For this review, take the finished solid that the model builds, in its own axes (mm). A direction names the side the tool comes from. Round coordinates to 2 decimals unless told otherwise and drop trailing zeros. Loops run counter-clockwise (first coordinate to the right, second up) from the corner with the lowest first, then second, coordinate; pieces in that order, holes last.
1) Wall thickness on L1, parallel to X at y = -1, z = -0.15; L2, parallel to X at y = -0.5, z = -0.4; L3, parallel to Z at x = 0.75, y = 0.75: over which ranges is each line inside the solid? List them lowest first.
2) Mouldability with a two-part tool opening along X and no side actions: class faces 3 (the flat face through (0, 4.674, -2)), 4 (the cylindrical face through (0.45, 0.5, 1.43)), 5 (the cylindrical face through (1.55, -3.15, -0.81)) as pulls with the +X half, pulls with the -X half, needs draft (parallel to the pull), parting line crosses it, or undercut.
3) Insertion check: pin 1 (3 mm diameter, centred on x = 0.5, y = 3.5, fed in from +Z); pin 2 (3 mm diameter, centred on x = 2, z = 2, fed in from -Y). Each pin has a flat end and moves straight along its axis. Give the tip position at first contact, or say it passes through.
4) Tool access review of faces 1 (the conical face through (1.9, 3.07, 0.42)), 2 (the flat face through (1.2, -3.8, -1.2)): name each direction out of +Z, -Z, +X, -X, +Y, -Y from which nothing blocks a thin tool from reaching the whole face with its end or side.
5) Take a section at B-B (x = 0). State the section outline as (y, z) points, then the cut area to 3 significant figures.
6) Take a section at A-A (z = 0). State the section outline as (x, y) points.
7) Take a section at C-C (y = 0.25). State the section outline as (x, z) points.
8) Take a section at D-D (z = -2.2). Give the number of separate pieces and of enclosed holes in the cut face, then the cut area to 3 significant figures.
```python
from build123d import *

# Parameters (mm, degrees)
ESQUISSE5_R             = 1.5
ENL_V_MAT_EXTRU_2_DEPTH = 10.476995662
CONG_2_R                = 0.5


with BuildPart() as part:
    # Esquisse1 → Révolution1 (revolve)
    with BuildSketch(Plane.XY):
        with BuildLine():
            Line((0, -3), (0, 3))
            ThreePointArc((0, 3), (3, 0), (0, -3))
        make_face()
    revolve(axis=Axis((0, 3, 0), (0, -1, 0)))

    # Esquisse4 → Révolution2 (revolve)
    with BuildSketch(Plane.XY, mode=Mode.PRIVATE) as r_volution2_sk:
        Polygon((1.75, 2.5), (2.5, 4.674281491), (0, 4.674281491), (0, 2.5), align=None)
    revolve(r_volution2_sk.sketch.rotate(Axis((0, -3.615713826, 0), (0, 1, 0)), 90), axis=Axis((0, -3.615713826, 0), (0, 1, 0)))

    # Esquisse6 → Révolution3 (revolve)
    with BuildSketch(Plane.XY, mode=Mode.PRIVATE) as r_volution3_sk:
        Polygon((0, -2.5), (1.75, -2.5), (1.75, -3.5), (2.703939201, -3.8), (0, -3.8), align=None)
    revolve(r_volution3_sk.sketch.rotate(Axis((0, -4.241210253, 0), (0, 1, 0)), 90), axis=Axis((0, -4.241210253, 0), (0, 1, 0)))

    # Esquisse5 → Enlèv. mat.-Extru.2 (cut, through all)
    with BuildSketch(Plane(origin=(0, 4.674281491, 0), x_dir=(1, 0, 0), z_dir=(0, 1, 0))):
        with Locations(Location((0, 0, 0), (0, 0, 270))):
            Circle(ESQUISSE5_R)
    extrude(amount=-ENL_V_MAT_EXTRU_2_DEPTH, mode=Mode.SUBTRACT)

    # Congé2
    # the kernel refuses this fillet: 0.5 mm, written as the material it takes off along each edge
    with BuildSketch(Plane(origin=(0, -2.5, 0), x_dir=(0, 0, -1), z_dir=(1, 0, 0))) as cong_2_piece_1:
        with BuildLine():
            CenterArc((1.25, -0.288584455), CONG_2_R, 0, 35.251664283)
            Line((1.75, -0.288584455), (1.75, 0))
            Line((1.75, 0), (1.658312395, 0))
        make_face()
    revolve(axis=Axis((0, -2.5, 0), (0, 1, 0)), mode=Mode.SUBTRACT)
    with BuildSketch(Plane(origin=(0, 2.5, 0), x_dir=(0, 0, -1), z_dir=(1, 0, 0))) as cong_2_piece_2:
        with BuildLine():
            CenterArc((1.359328414, 0.400760002), CONG_2_R, 306.724501908, 34.244057167)
            Line((1.831998303, 0.237716523), (1.75, 0))
            Line((1.75, 0), (1.658312395, 0))
        make_face()
    revolve(axis=Axis((0, 2.5, 0), (0, 1, 0)), mode=Mode.SUBTRACT)


solid = part.part
```
Response:
1. L1: x = -2.82 to -1.49, 1.49 to 2.82
1. L2: x = -2.93 to -1.45, 1.45 to 2.93
1. L3: z = -2.81 to -1.3, 1.3 to 2.81
2. face 3: needs draft
2. face 4: undercut
2. face 5: parting line crosses it
3. pin 1: stops at z = 2.5
3. pin 2: stops at y = -3.8
4. face 1: none
4. face 2: +Z, -Z, +X, -X, -Y
5. outline: (-3.8, -2.7) - (-3.5, -1.75) - (-2.79, -1.75) arc R0.5 ccw to (-2.5, -1.66) arc R3 ccw to (2.5, -1.66) arc R0.5 ccw to (2.74, -1.83) - (4.67, -2.5) - (4.67, -1.5) - (-3.8, -1.5) - close; (-3.8, 1.5) - (4.67, 1.5) - (4.67, 2.5) - (2.74, 1.83) arc R0.5 ccw to (2.5, 1.66) arc R3 ccw to (-2.5, 1.66) arc R0.5 ccw to (-2.79, 1.75) - (-3.5, 1.75) - (-3.8, 2.7) - close
5. area: 14.6 mm2
6. outline: (-2.7, -3.8) - (-1.5, -3.8) - (-1.5, 4.67) - (-2.5, 4.67) - (-1.83, 2.74) arc R0.5 ccw to (-1.66, 2.5) arc R3 ccw to (-1.66, -2.5) arc R0.5 ccw to (-1.75, -2.79) - (-1.75, -3.5) - close; (1.5, -3.8) - (2.7, -3.8) - (1.75, -3.5) - (1.75, -2.79) arc R0.5 ccw to (1.66, -2.5) arc R3 ccw to (1.66, 2.5) arc R0.5 ccw to (1.83, 2.74) - (2.5, 4.67) - (1.5, 4.67) - close
7. outline: circle Ø5.98 at (0, 0); hole circle Ø3 at (0, 0)
8. separate pieces: 3
8. enclosed holes: 0
8. area: 14.8 mm2
